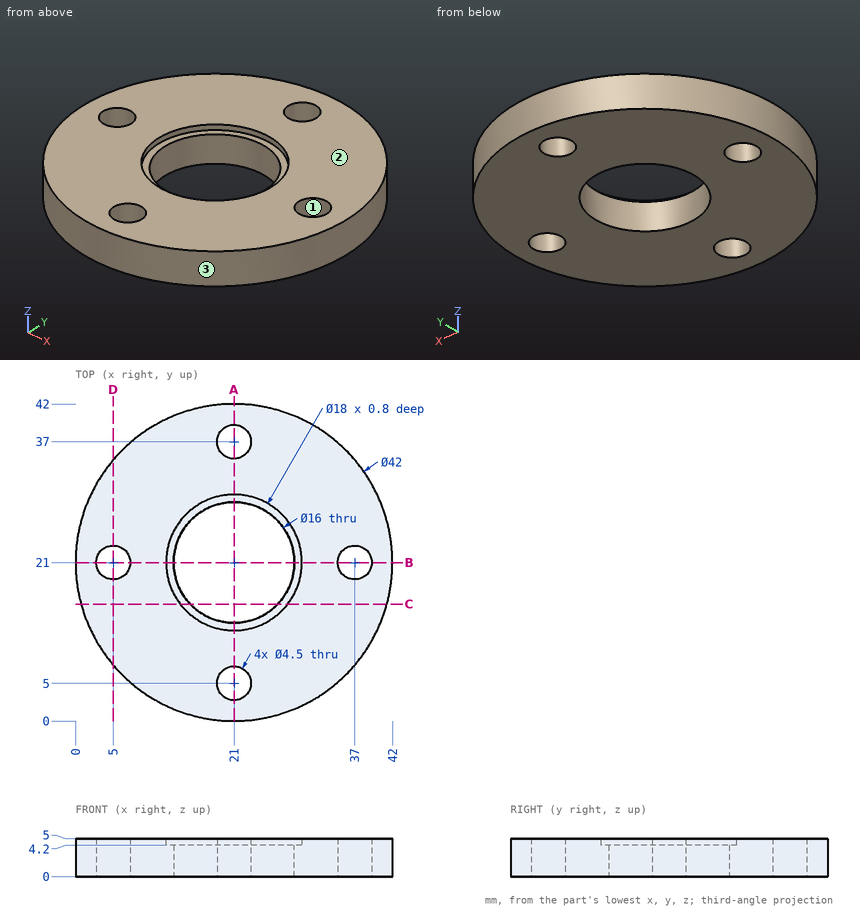
Print and shaded views of the part. All mm, measured from the part's lowest x, y and z. Coordinates: 2 decimals unless noted, no trailing zeros. Order: outer loops, then holes, each group sorted by start corner. A loop starts at its lowest first (then second) coordinate and runs counter-clockwise, first axis right, second up. Notation, with made-up numbers: (-3.75, 58.25) -> (18.25, 58.25) arc R13 ccw to (18.25, 82.25) -> close; hole circle Ø9 at (65.25, -1). An arc over 180 degrees is marked (long way). Use one line per item in the form item = value. Start each with the question number.
1) Band-saw the part on C-C on y = 15.5. Give the cut face in (x, z), then the cut area to 3 significant figures.
2) Drop flat-ended pins along their axis: pin 1 (1.5 mm diameter, centred on y = 19.5, z = 1.5, fed in from -X); pin 2 (1 mm diameter, centred on x = 7.5, z = 2, fed in from -Y); pin 3 (14.5 mm diameter, centred on x = 22, y = 21.5, fed in from +Z). Give the stop position or say it passes through.
3) Drill centre lines: L1, parallel to Y at x = 21, z = 3; L2, parallel to X at y = 20, z = 2.45; L3, parallel to X at y = 38, z = 1.8. Where is each one in solid material? Low to high. Write a range as [from, to].
4) Pull direction X, two halves, no side cores. Call the marked faces 1, 2 and 3: +X half, -X half, draft (parallel to the pull), parting line (faces both ways), or undercut.
5) Band-saw the part on D-D on x = 5. Give the cut face in (y, z), then the cut area to 3 significant figures.
6) Band-saw the part on A-A on x = 21. Give the cut face in (y, z).
Entries:
q1.outline = (0.73, 0) -> (15.19, 0) -> (15.19, 4.2) -> (13.88, 4.2) -> (13.88, 5) -> (0.73, 5) -> close; (26.81, 0) -> (41.27, 0) -> (41.27, 5) -> (28.12, 5) -> (28.12, 4.2) -> (26.81, 4.2) -> close
q1.area = 142 mm2
q2.pin_1 = 0.01
q2.pin_2 = 4.51
q2.pin_3 = 4.2
q3.L1 = [0, 2.75], [7.25, 13], [29, 34.75], [39.25, 42]
q3.L2 = [0.02, 2.98], [7.02, 13.06], [28.94, 34.98], [39.02, 41.98]
q3.L3 = [8.67, 18.98], [23.02, 33.33]
q4.face_1 = undercut
q4.face_2 = draft
q4.face_3 = parting line
q5.outline = (7.4, 0) -> (18.75, 0) -> (18.75, 5) -> (7.4, 5) -> close; (23.25, 0) -> (34.6, 0) -> (34.6, 5) -> (23.25, 5) -> close
q5.area = 114 mm2
q6.outline = (0, 0) -> (2.75, 0) -> (2.75, 5) -> (0, 5) -> close; (7.25, 0) -> (13, 0) -> (13, 4.2) -> (12, 4.2) -> (12, 5) -> (7.25, 5) -> close; (29, 0) -> (34.75, 0) -> (34.75, 5) -> (30, 5) -> (30, 4.2) -> (29, 4.2) -> close; (39.25, 0) -> (42, 0) -> (42, 5) -> (39.25, 5) -> close
